from build123d import *

# Parameters (mm, degrees)
SKETCH1_R           = 1.375
BOSS_EXTRUDE1_DEPTH = 6
BOSS_EXTRUDE2_START = -13.125
SKETCH9_W           = 3.5
SKETCH9_H           = 3
BOSS_EXTRUDE2_DEPTH = 7.26
BOSS_EXTRUDE3_START = -3.5
SKETCH10_W          = 3
SKETCH10_H          = 3
BOSS_EXTRUDE3_DEPTH = 23.25
SKETCH11_W          = 3
SKETCH11_H          = 3
BOSS_EXTRUDE4_DEPTH = 5
FILLET1_R           = 2.5
FILLET2_R           = 1
FILLET3_R           = 3
CUT_EXTRUDE1_REACH  = 51.544
SKETCH12_R          = 1


with BuildPart() as part:
    # Sketch1 → Boss-Extrude1 (new body)
    with BuildSketch(Plane(origin=(0, 0, 0), x_dir=(0, 1, 0), z_dir=(0, 0, 1))):
        with BuildLine():
            Line((0, 2.875), (7, 2.875))
            Line((7, 2.875), (7, -2.875))
            Line((7, -2.875), (0, -2.875))
            ThreePointArc((0, -2.875), (-2.875, 0), (0, 2.875))
        make_face()
        with Locations(Location((0, 0, 0), (0, 0, 270))):
            Circle(SKETCH1_R, mode=Mode.SUBTRACT)
    extrude(amount=BOSS_EXTRUDE1_DEPTH)

    # Sketch2 → Loft1 section 0
    with BuildSketch(Plane(origin=(0, 0, 0), x_dir=(1, 0, 0), z_dir=(0, 0, -1))):
        with BuildLine():
            Line((0.875, -7), (-2.875, -7))
            Line((-2.875, -7), (-2.875, -3.5))
            Line((-2.875, -3.5), (0.875, -3.5))
            Line((0.875, -3.5), (0.875, -7))
        make_face()
    # Sketch8 → Loft1 section 1
    with BuildSketch(Plane(origin=(0, 0, -37.5), x_dir=(-1, 0, 0), z_dir=(0, 0, -1))):
        with BuildLine():
            Line((2.375, 3.5), (2.375, 7))
            Line((2.375, 7), (6.125, 7))
            Line((6.125, 7), (6.125, 3.5))
            Line((6.125, 3.5), (2.375, 3.5))
        make_face()
    loft()

    # Sketch9 → Boss-Extrude2 (add)
    with BuildSketch(Plane.YZ.offset(BOSS_EXTRUDE2_START)):
        with Locations((5.25, -36)):
            Rectangle(SKETCH9_W, SKETCH9_H)
    extrude(amount=BOSS_EXTRUDE2_DEPTH)

    # Sketch10 → Boss-Extrude3 (add)
    with BuildSketch(Plane(origin=(0, 7, 0), x_dir=(-1, 0, 0), z_dir=(0, 1, 0)).offset(BOSS_EXTRUDE3_START)):
        with Locations((11.625, -36)):
            Rectangle(SKETCH10_W, SKETCH10_H)
    extrude(amount=-BOSS_EXTRUDE3_DEPTH)

    # Sketch11 → Boss-Extrude4 (add)
    with BuildSketch(Plane.XY.offset(-34.5)):
        with Locations((-11.625, -18.25)):
            Rectangle(SKETCH11_W, SKETCH11_H)
    extrude(amount=BOSS_EXTRUDE4_DEPTH)

    # Fillet1
    # the kernel refuses this fillet: 2.5 mm, written as the material it adds along each edge
    with BuildSketch(Plane(origin=(0.875, 3.5, 0), x_dir=(-0.08634300732914678, 0, -0.9962654691824658), z_dir=(0, 1, 0))) as fillet1_piece_1:
        with BuildLine():
            CenterArc((2.275267243, -2.5), FILLET1_R, 90, 78.288278187)
            Line((-0.172686015, -1.992530938), (0, 0))
            Line((0, 0), (2.275267243, 0))
        make_face()
    extrude(amount=3.5)
    # the kernel refuses this fillet: 2.5 mm, written as the material it takes off along each edge
    with BuildSketch(Plane(origin=(-19.375, -19.75, -37.5), x_dir=(0, 0, 1), z_dir=(1, 0, 0))) as fillet1_2_piece_1:
        with BuildLine():
            CenterArc((FILLET1_R, -FILLET1_R), FILLET1_R, 90, 90)
            Line((0, -FILLET1_R), (0, 0))
            Line((0, 0), (FILLET1_R, 0))
        make_face()
    extrude(amount=15.5, mode=Mode.SUBTRACT)
    with BuildSketch(Plane(origin=(-2.375, -2.231761645, -37.5), x_dir=(-1, 0, 0), z_dir=(0, 1, 0))) as fillet1_2_piece_2:
        with BuildLine():
            CenterArc((FILLET1_R * 0.917081863151, FILLET1_R), FILLET1_R, 184.953257478, 85.046742522)
            Line((-FILLET1_R * 0.0791836060315, FILLET1_R * 0.913656992671), (0, 0))
            Line((0, 0), (FILLET1_R * 0.917081863151, 0))
        make_face()
    extrude(amount=14.963523289, mode=Mode.SUBTRACT)
    with BuildSketch(Plane(origin=(-13.125, 7, -43.75), x_dir=(0, -1, 0), z_dir=(0, 0, 1))) as fillet1_2_piece_3:
        with BuildLine():
            CenterArc((FILLET1_R, FILLET1_R), FILLET1_R, 180, 90)
            Line((0, FILLET1_R), (0, 0))
            Line((0, 0), (FILLET1_R, 0))
        make_face()
    extrude(amount=15.5, mode=Mode.SUBTRACT)

    # Fillet2
    fillet2_edges = [part.edges().sort_by_distance(p)[0] for p in [
        (0, 7, 6),
        (-5.865, 5.25, -34.5),
        (-11.625, -16.75, -34.5),
        (-11.625, -16.75, -29.5),
        (-13.125, -18.25, -29.5),
        (-11.625, -19.75, -29.5),
        (-10.125, -18.25, -29.5),
    ]]
    fillet(fillet2_edges, radius=FILLET2_R)

    # Fillet3
    fillet3_edges = [part.edges().sort_by_distance(p)[0] for p in [
        (-10.125, 3.5, -36),
    ]]
    fillet(fillet3_edges, radius=FILLET3_R)

    # Sketch12 → Cut-Extrude1 (cut, up to next)
    with BuildSketch(Plane(origin=(0, 0, -37.5), x_dir=(1, 0, 0), z_dir=(0, 0, -1)), mode=Mode.PRIVATE) as cut_extrude1_sk1:
        with Locations(Location((-10.819543648, -4.444543648, 0), (0, 0, 180))):
            Circle(SKETCH12_R)
    cut_extrude1_tool1 = extrude(cut_extrude1_sk1.sketch, amount=-CUT_EXTRUDE1_REACH, mode=Mode.PRIVATE) & part.part
    add(cut_extrude1_tool1.solids().sort_by_distance((-10.819544, 4.444544, -37.5))[0], mode=Mode.SUBTRACT)


solid = part.part
Check sheet for the modelled part. Datum: model origin and axes. Units: mm. A direction names the side the tool comes from. Round coordinates to 2 decimals unless told otherwise and drop trailing zeros. Order: outer loops, then holes, each group sorted by start corner. A loop starts at its lowest first (then second) coordinate and runs counter-clockwise, first axis right, second up.
Q1. Cross-section at C-C, the plane x = 0. Enter the section's corners in (y, z) (3 decimals).
Filled sheet:
outline: (-2.875, 0) - (-1.375, 0) - (-1.375, 6) - (-2.875, 6) - close; (1.375, 0) - (3.5, 0) - (3.5, -10.096) - (7, -10.096) - (7, 5) arc R1 ccw to (6, 6) - (1.375, 6) - close
Q2. Cross-section at D-D, the plane y = -0.5. Enter the section's corners in (x, z) (3 decimals), plus the area to 3 significant figures.
Filled sheet:
outline: (-13.125, -37.5) - (-10.125, -37.5) - (-10.125, -34.5) - (-13.125, -34.5) - close; (-2.831, 0) - (-1.281, 0) - (-1.281, 6) - (-2.831, 6) - close; (1.281, 0) - (2.831, 0) - (2.831, 6) - (1.281, 6) - close
area: 27.6 mm2
Q3. Cross-section at A-A, the plane y = 2.5. Enter the section's corners in (x, z) (3 decimals), plus the area to 3 significant figures.
Filled sheet:
outline: (-13.125, -37.5) - (-9.361, -37.5) - (-9.361, -34.5) - (-13.125, -34.5) - close; (-2.875, 0) - (2.875, 0) - (2.875, 6) - (-2.875, 6) - close
area: 45.8 mm2
Q4. Set-up check for faces 1 (the face through (-3, 3.5, -19)), 2 (the face through (-10.125, -10, -36)), 3 (the face through (-12, -16.75, -32)), 4 (the face through (-11, -2, -34.5)): record each of +Z, -Z, +X, -X, +Y, -Y from which the full face is reachable in a straight line by a thin tool's end or side.
Filled sheet:
face 1: -Z, +X, -Y
face 2: +Z, -Z, +X, -Y
face 3: +Z, +X, -X, +Y
face 4: +Z, -X, +Y
Q5. Cross-section at B-B, the plane z = 3. Enter the section's corners in (x, y) (3 decimals), plus the area to 3 significant figures.
Filled sheet:
outline: (-2.875, 0) arc R2.875 ccw to (2.875, 0) - (2.875, 7) - (-2.875, 7) - close; hole circle Ø2.75 at (0, 0)
area: 47.3 mm2
Q6. Depth check by flat-ended pin: P1, Ø3.5, axis at y = -11.5, z = -33, coming from the +X side (3 decimals); P2, Ø5, axis at x = -5.5, y = -7, coming from the -Z side; P3, Ø3.5, axis at x = -12, z = -31.5, coming from the +Y side; P4, Ø4.5, axis at x = 1.5, y = 0, coming from the -Z side. Enter the tip coordinate at first touch or a pass-through.
Filled sheet:
P1: stops at x = -10.125
P2: passes through
P3: stops at y = -16.75
P4: stops at z = 0
Q7. Scan lines: L1, parallel to Y at x = 0, z = 2 (3 decimals); L2, parallel to Y at x = -3.5, z = -12; L3, parallel to Z at x = -10.5, y = -8. Record each from-to range of solid material in increasing order.
Filled sheet:
L1: y = -2.875 to -1.375, 1.375 to 7
L2: y = 3.5 to 7
L3: z = -37.5 to -34.5
